```python
from build123d import *

# Parameters (mm, degrees)
F1_DEPTH = 20
F3_DEPTH = 20
F5_DEPTH = 12


with BuildPart() as f1:
    # F0 (on Top) → F1 (new body)
    with BuildSketch(Plane.XY):
        with BuildLine():
            Line((76.790496, 19.411137), (-1.14431, 11.945315))
            ThreePointArc((-1.14431, 11.945315), (-12, 0), (-1.14431, -11.945315))
            Line((-1.14431, -11.945315), (76.790496, -19.411137))
            ThreePointArc((76.790496, -19.411137), (98.15, 0), (76.790496, 19.411137))
        make_face()
    extrude(amount=F1_DEPTH)

    # F2 (on face) → F3 (join)
    with BuildSketch(Plane.XY.offset(20)):
        with BuildLine():
            ThreePointArc((76.790496, -19.411137), (91.76468, -14.431049), (98.15, 0))
            ThreePointArc((98.15, 0), (91.76468, 14.431049), (76.790496, 19.411137))
            ThreePointArc((76.790496, 19.411137), (59.15, 0), (76.790496, -19.411137))
        make_face()
    extrude(amount=F3_DEPTH)

    # F4 (on face) → F5 (join)
    with BuildSketch(Plane.XY.offset(20)):
        with BuildLine():
            ThreePointArc((-1.14431, -11.945315), (8.070572, -8.880645), (12, 0))
            ThreePointArc((12, 0), (8.070572, 8.880645), (-1.14431, 11.945315))
            ThreePointArc((-1.14431, 11.945315), (-12, 0), (-1.14431, -11.945315))
        make_face()
    extrude(amount=F5_DEPTH)


solid = f1.part
```
Could you check a few things on this model? Use its own coordinates, in mm. A direction names the side the tool comes from. Give positions to 0.01 mm unless a question says otherwise; leave off trailing zeros. Loops run counter-clockwise (first coordinate to the right, second up) from the corner with the lowest first, then second, coordinate; pieces in that order, holes last. Notation, with made-up numbers: (82.25, -39.5) - (125.25, -39.5) arc R9 ccw to (125.25, -25.5) - close; hole circle Ø8 at (-14.75, 15). An arc over 180 degrees is marked (long way). Answer in a Markdown table with one row per item. Add a question column.
Q1. If we section it at B-B (x = 66): List the corners of the cut face in (y, z) for me.
Q2. For pin 1 (12 mm diameter, centred on y = -15, z = 10, fed in from +X); pin 2 (4 mm diameter, centred on y = -9.5, z = 16, fed in from -X); pin 3 (7 mm diameter, centred on x = -2.5, y = 1, fed in from +Z), each with a flat end and sliding along its axis, tell me the tip position at first contact or that it passes through.
Q3. Please list where these lines run through material, in increasing order: L1, parallel to Z at x = 47.5, y = -11.5; L2, parallel to X at y = 6, z = 30; L3, parallel to Y at x = 20, z = 7.5. Write a range as from..to.
Q4. If we section it at C-C (z = 15.5): List the corners of the cut face in (x, y) for me.
Q5. If we section it at A-A (y = -5.5): List the corners of the cut face in (x, z) for me.
Q6. Which directions (+Z, -Z, +X, -X, +Y, -Y) give clear straight access to the entire face, cutting with the end or side of a thin tool? Please do faces 1 (the face through (0, 0, 32)), 2 (the face through (42, 0, 0)).
Q7. If we section it at D-D (y = 3): List the corners of the cut face in (x, z) for me, plus the area to 3 significant figures.
The answers:
| question | item | result |
|---|---|---|
| 1 | outline | (-18.38, 0) - (18.38, 0) - (18.38, 20) - (14.84, 20) - (14.84, 40) - (-14.84, 40) - (-14.84, 20) - (-18.38, 20) - close |
| 2 | pin 1 | stops at x = 95.95 |
| 2 | pin 2 | stops at x = -9.37 |
| 2 | pin 3 | stops at z = 32 |
| 3 | L1 | z = 0..20 |
| 3 | L2 | x = -10.39..10.39, 60.1..97.2 |
| 3 | L3 | y = -13.97..13.97 |
| 4 | outline | (-1.14, -11.95) - (76.79, -19.41) arc R19.5 ccw (long way) to (76.79, 19.41) - (-1.14, 11.95) arc R12 ccw to start |
| 5 | outline | (-10.67, 0) - (97.36, 0) - (97.36, 40) - (59.94, 40) - (59.94, 20) - (10.67, 20) - (10.67, 32) - (-10.67, 32) - close |
| 6 | face 1 | +Z, -X, +Y, -Y |
| 6 | face 2 | -Z, +X, -X, +Y, -Y |
| 7 | outline | (-11.62, 0) - (97.92, 0) - (97.92, 40) - (59.38, 40) - (59.38, 20) - (11.62, 20) - (11.62, 32) - (-11.62, 32) - close |
| 7 | area | 3,240 mm^2 |
